Study the drawing (mm; zero at the part's minimum x, y, z) and answer. Coordinates: 2 decimals unless noted, no trailing zeros. Order: outer loops, then holes, each group sorted by start corner. A loop starts at its lowest first (then second) coordinate and runs counter-clockwise, first axis right, second up. Notation, with made-up numbers: (-6, -23.5) -> (16, -23.5) arc R9 cw to (16, -17.5) -> close; hole circle Ø6 at (-2, -23.75). An arc over 180 degrees is marked (long way). Put each result on its own line as item: value. Start each with the question number.
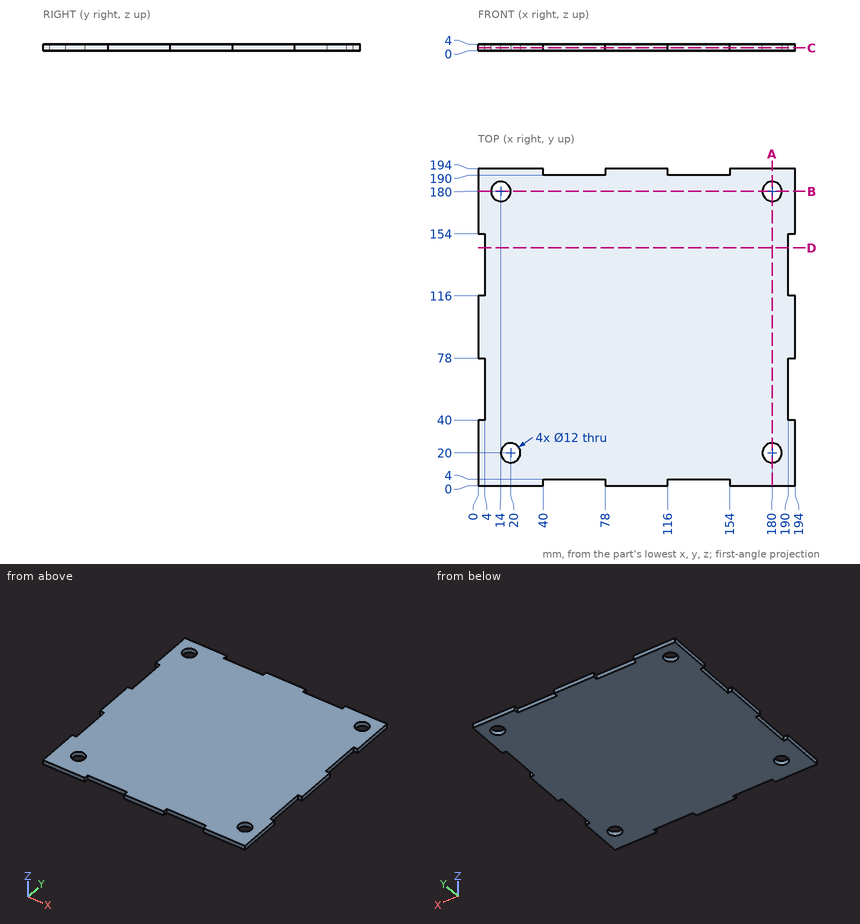
(1) Find the intervals of material crossed by L1, parallel to Y at x = 180, z = 3.1; L2, parallel to X at y = 179.5, z = 1.5; L3, parallel to X at y = 24, z = 2, in increasing order.
(2) The part is cut by section C-C on z = 1.65. Count the separate pieces of the cut face and the enclosed holes in it, plus the area to 3 significant figures.
(3) The part is cut by section B-B on y = 180. Determine the outline of the cut face in (x, z), plus the area to 3 significant figures.
(4) The part is cut by section A-A on x = 180. Determine the outline of the cut face in (y, z), plus the area to 3 significant figures.
(5) The part is cut by section D-D on y = 145.5. Determine the outline of the cut face in (x, z).
(6) Each of these flat-tipped pins is pushed along its axis until it touches: P1, Ø2, axis at y = 192, z = 1.5, coming from the -X side; P2, Ø2, axis at x = 119, z = 2.5, coming from the -Y side. Where does it stop, or does it pass through?
Worked out:
1. L1: 0 to 14, 26 to 174, 186 to 194
1. L2: 0 to 8.02, 19.98 to 174.02, 185.98 to 194
1. L3: 0 to 15.53, 24.47 to 175.53, 184.47 to 194
2. separate pieces: 1
2. enclosed holes: 4
2. area: 36,000 mm2
3. outline: (0, 0) -> (8, 0) -> (8, 4) -> (0, 4) -> close; (20, 0) -> (174, 0) -> (174, 4) -> (20, 4) -> close; (186, 0) -> (194, 0) -> (194, 4) -> (186, 4) -> close
3. area: 680 mm2
4. outline: (0, 0) -> (14, 0) -> (14, 4) -> (0, 4) -> close; (26, 0) -> (174, 0) -> (174, 4) -> (26, 4) -> close; (186, 0) -> (194, 0) -> (194, 4) -> (186, 4) -> close
4. area: 680 mm2
5. outline: (4, 0) -> (190, 0) -> (190, 4) -> (4, 4) -> close
6. P1: x = 0
6. P2: y = 4
